```python
from build123d import *

# Parameters (mm, degrees)
F1_DEPTH      = 30
F1_DEPTH_BACK = 15
F3_DEPTH      = 25
F4_W          = 5
F4_H          = 5
F5_DEPTH      = 2
F6_SIZE2      = 1
F6_SIZE       = 1


with BuildPart() as f1:
    # F0 (on Front) → F1 (new body, two sides)
    with BuildSketch(Plane.XZ) as f1_sk:
        with BuildLine():
            Line((0, -1), (40, -1))
            Line((40, -1), (40, 1))
            Line((40, 1), (0, 1))
            Line((0, 1), (0, 21))
            Line((0, 21), (-2, 21))
            Line((-2, 21), (-2, 1))
            ThreePointArc((-2, 1), (-1.414214, -0.414214), (0, -1))
        make_face()
    extrude(amount=F1_DEPTH)
    extrude(f1_sk.sketch, amount=-F1_DEPTH_BACK)

    # F2 (on face) → F3 (cut)
    with BuildSketch(Plane.XY.offset(1)):
        with BuildLine():
            Line((35.75, 11.651385), (7.75, 11.651385))
            ThreePointArc((7.75, 11.651385), (5.5, 9.401385), (7.75, 7.151385))
            Line((7.75, 7.151385), (35.75, 7.151385))
            ThreePointArc((35.75, 7.151385), (38, 9.401385), (35.75, 11.651385))
        make_face()
        with BuildLine():
            Line((21.75, -6.848615), (21.75, -21.848615))
            ThreePointArc((21.75, -21.848615), (25.75, -25.848615), (29.75, -21.848615))
            Line((29.75, -21.848615), (29.75, -6.848615))
            ThreePointArc((29.75, -6.848615), (25.75, -2.848615), (21.75, -6.848615))
        make_face()
        with BuildLine():
            Line((35.75, 4.651385), (7.75, 4.651385))
            ThreePointArc((7.75, 4.651385), (5.5, 2.401385), (7.75, 0.151385))
            Line((7.75, 0.151385), (35.75, 0.151385))
            ThreePointArc((35.75, 0.151385), (38, 2.401385), (35.75, 4.651385))
        make_face()
    extrude(amount=-F3_DEPTH, mode=Mode.SUBTRACT)

    # F4 (on face) → F5 (join, through all)
    with BuildSketch(Plane.XY.offset(1)):
        with Locations((42.5, 0)):
            Rectangle(F4_W, F4_H)
    extrude(amount=-F5_DEPTH)

    # F6
    f6_edges = [f1.edges().sort_by_distance(p)[0] for p in [
        (-1, 15, 21),
        (-1, -30, 21),
        (40, -30, 0),
        (40, 15, 0),
        (45, 2.5, 0),
        (45, -2.5, 0),
    ]]
    chamfer(f6_edges, length=F6_SIZE, length2=F6_SIZE2)


solid = f1.part
```
Here's how the part is built. I have some questions about the finished solid (model axes, mm). A direction names the side the tool comes from. Round coordinates to 2 decimals unless told otherwise and drop trailing zeros. Order: outer loops, then holes, each group sorted by start corner. A loop starts at its lowest first (then second) coordinate and runs counter-clockwise, first axis right, second up. Notation, with made-up numbers: M 36.25,21.25 L 86.25,21.25 A37 cw 86.25,60.25 Z; hole C -28,49 d9. An arc over 180 degrees is marked long. Answer in a Markdown table with one row per item.
Item 1: I'm going to push flat-ended pins straight in: pin 1 (3 mm diameter, centred on y = -17.5, z = 8.5, fed in from +X); pin 2 (1 mm diameter, centred on x = 6, y = -6.5, fed in from +Z); pin 3 (0.6 mm diameter, centred on y = -16, z = 0.5, fed in from +X); pin 4 (10 mm diameter, centred on x = 31, z = 10.5, fed in from +Y). Where does each tip first touch, or does it pass through?
A:
| item | result |
|---|---|
| pin 1 | stops at x = 0 |
| pin 2 | stops at z = 1 |
| pin 3 | stops at x = 40 |
| pin 4 | passes through |
Item 2: Imagine slicing it at C-C, the plane x = 16.5. Write out the boundary of the cut face in (y, z).
A:
| item | result |
|---|---|
| outline | M -30,-1 L 0.15,-1 L 0.15,1 L -30,1 Z; M 4.65,-1 L 7.15,-1 L 7.15,1 L 4.65,1 Z; M 11.65,-1 L 15,-1 L 15,1 L 11.65,1 Z |
Item 3: Imagine slicing it at B-B, the plane x = 25.75. Write out the boundary of the cut face in (y, z), and give its area (3 significant figures).
A:
| item | result |
|---|---|
| outline | M -30,-1 L -25.85,-1 L -25.85,1 L -30,1 Z; M -2.85,-1 L 0.15,-1 L 0.15,1 L -2.85,1 Z; M 4.65,-1 L 7.15,-1 L 7.15,1 L 4.65,1 Z; M 11.65,-1 L 15,-1 L 15,1 L 11.65,1 Z |
| area | 26.0 mm2 |
Item 4: Thinking about a two-plate mould opening in Y: for faces 5 (the face through (25.84, -2.85, 0.01)), 6 (the face through (-2, -8, 11)), 7 (the face through (14, -30, 0)), which applies, +Y half, -Y half, draft (parallel to the pull), parting line (faces both ways), or undercut?
A:
| item | result |
|---|---|
| face 5 | undercut |
| face 6 | draft |
| face 7 | -Y half |
Item 5: Imagine slicing it at A-A, the plane y = -20. Write out the boundary of the cut face in (x, z), and give its area (3 significant figures).
A:
| item | result |
|---|---|
| outline | M -2,1 A2 ccw 0,-1 L 21.75,-1 L 21.75,1 L 0,1 L 0,21 L -2,21 Z; M 29.75,-1 L 40,-1 L 40,1 L 29.75,1 Z |
| area | 107 mm2 |
Item 6: If I drill on L1, parallel to X at y = -1, z = 5.75; L2, parallel to Z at x = 7, y = -2; L3, parallel to X at y = -10.5, z = 0.75, over which ranges is the centre line in solid material (lowest first)? Write a range as from..to.
A:
| item | result |
|---|---|
| L1 | x = -2..0 |
| L2 | z = -1..1 |
| L3 | x = -1.98..21.75, 29.75..40 |
Item 7: For faces 1 (the face through (0, -8, 11)), 2 (the face through (5.5, 9.45, 0.01)), 3 (the face through (42, 2.5, 0)), 4 (the face through (40, -16, 0)), which set-ups out of +Z, -Z, +X, -X, +Y, -Y let a thin tool reach every point of the face, with its end or its side?
A:
| item | result |
|---|---|
| face 1 | +Z, +X, +Y, -Y |
| face 2 | +Z, -Z |
| face 3 | +Z, -Z, +X, +Y |
| face 4 | +Z, -Z, +X, -Y |
Item 8: Imagine slicing it at D-D, the plane z = 12. Write out the boundary of the cut face in (x, y).
A:
| item | result |
|---|---|
| outline | M -2,-30 L 0,-30 L 0,15 L -2,15 Z |
